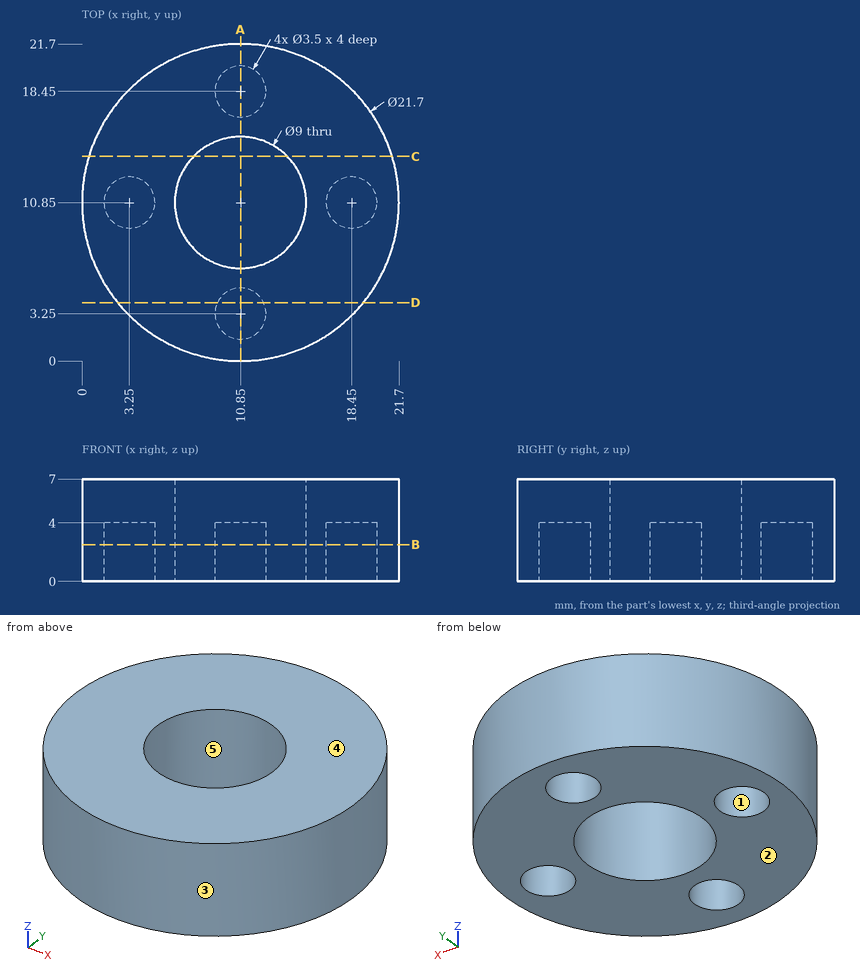
Geometry check sheet. Reference: drawing and pictorial views, mm from the part's lowest x, y, z. A direction names the side the tool comes from. Coordinates: 2 decimals unless noted, no trailing zeros. Order: outer loops, then holes, each group sorted by start corner. A loop starts at its lowest first (then second) coordinate and runs counter-clockwise, first axis right, second up. Notation, with made-up numbers: (42, -1) -> (82, -1) arc R3 ccw to (82, 4) -> close; hole circle Ø1 at (62.25, 81.5). An arc over 180 degrees is marked (long way). Write item = value, one per line. Start each with the question number.
1) Mould release check, pull along Y, two halves, no side actions. Record for the marked faces 3, 4 and 5: +Y half, -Y half, draft (parallel to the pull), parting line (faces both ways), or undercut.
2) Cross-section at C-C (y = 14). Enter the section's corners in (x, z).
3) Cross-section at D-D (y = 4). Enter the section's corners in (x, z).
4) Material ranges on L1, parallel to Y at x = 10.85, z = 1.1; L2, parallel to Y at x = 11, z = 5.5; L3, parallel to Y at x = 14, z = 5, recorded low to high.
5) Access from +Z, -Z, +X, -X, +Y, -Y to the whole of each face (thin tool, end or side, straight path). Record for the marked faces 1 and 2.
6) Cross-section at B-B (z = 2.5). Enter the section's corners in (x, y).
7) Cross-section at A-A (x = 10.85). Enter the section's corners in (y, z).
8) Go/stop test with flat-tipped pins: P1, Ø4, axis at x = 10.5, y = 3.5, coming from the -Z side; P2, Ø1, axis at x = 11, y = 19, coming from the -Z side; P3, Ø4, axis at y = 5.5, z = 2.5, coming from the +X side. Record where each tip stops, or that it passes through.
Ans:
q1.face_3 = parting line
q1.face_4 = draft
q1.face_5 = undercut
q2.outline = (0.47, 0) -> (7.64, 0) -> (7.64, 7) -> (0.47, 7) -> close; (14.06, 0) -> (21.23, 0) -> (21.23, 7) -> (14.06, 7) -> close
q3.outline = (2.44, 0) -> (9.27, 0) -> (9.27, 4) -> (12.43, 4) -> (12.43, 0) -> (19.26, 0) -> (19.26, 7) -> (2.44, 7) -> close
q4.L1 = 0 to 1.5, 5 to 6.35, 15.35 to 16.7, 20.2 to 21.7
q4.L2 = 0 to 6.35, 15.35 to 21.7
q4.L3 = 0.47 to 7.64, 14.06 to 21.23
q5.face_1 = -Z
q5.face_2 = -Z, +X, -X, +Y, -Y
q6.outline = circle Ø21.7 at (10.85, 10.85); hole circle Ø3.5 at (3.25, 10.85); hole circle Ø9 at (10.85, 10.85); hole circle Ø3.5 at (10.85, 3.25); hole circle Ø3.5 at (10.85, 18.45); hole circle Ø3.5 at (18.45, 10.85)
q7.outline = (0, 0) -> (1.5, 0) -> (1.5, 4) -> (5, 4) -> (5, 0) -> (6.35, 0) -> (6.35, 7) -> (0, 7) -> close; (15.35, 0) -> (16.7, 0) -> (16.7, 4) -> (20.2, 4) -> (20.2, 0) -> (21.7, 0) -> (21.7, 7) -> (15.35, 7) -> close
q8.P1 = 0
q8.P2 = 4
q8.P3 = 21.17
